Design review of the part built by this model. Coordinates are the model's own, in mm. Give positions to 0.01 mm unless a question says otherwise; leave off trailing zeros. Write each loop counter-clockwise with the first axis right and the second up, starting at its lowest first coordinate (ties: lowest second). Pieces come first, ordered by that corner, then holes. Notation, with made-up numbers: (83.5, 62.25) -> (140.5, 62.25) arc R20 ccw to (140.5, 79.25) -> close; hole circle Ø3 at (-36.5, 32.5). An arc over 180 degrees is marked (long way). Use CSV: the item, a comma, the result in double quotes.
Autodesk Inventor part; units mm, degrees
ref_plane "Work Plane1" through (167.5, 74.771, 0) normal (0.7444, -0.6677, 0) x (0.6677, 0.7444, 0)
ref_plane "Work Plane2" through (0, 0, 0) normal (0, -1, 0) x (1, 0, 0)
ref_plane "YZ Plane" through (0, 0, 0) normal (1, 0, 0) x (0, 1, 0)
sketch "Sketch1" plane through (0, 0, 0) normal (0, 0, 1) x (1, 0, 0)
  circle A0 centre (0, 225) radius 225 construction
  circle A1 centre (0, 225) radius 220 construction
  line L0 (0, 5) -> (0, 0)
  arc A2 (0, 0) -> (167.5, 74.771) centre (0, 225) ccw
  line L1 (167.5, 74.771) -> (163.7778, 78.1094)
  arc A3 (0, 5) -> (163.7778, 78.1094) centre (0, 225) ccw
  dimension "d0" = 450
  dimension "d1" = 5
  dimension "d2" = 5
  dimension "d3" = 167.5
extrude "Extrusion1" add sketch "Sketch1" along normal blind 75
ref_plane "Work Plane1" through (167.5, 74.771, 0) normal (0.7444, -0.6677, 0) x (0.6677, 0.7444, 0)
sketch "Sketch2" plane through (167.5, 74.771, 0) normal (0.7444, -0.6677, 0) x (0.6677, 0.7444, 0)
  circle A0 centre (-5, 47.5) radius 3
  circle A1 centre (-5, 27.5) radius 3
  line L0 (0, 0) -> (-167.5, 0)
  line L1 (0, 0) -> (0, 75)
  line L2 (-167.5, 75) -> (0, 75)
  line L3 (-167.5, 0) -> (-167.5, 75)
  dimension "d6" = 6
  dimension "d7" = 6
  dimension "d8" = 5
  dimension "d9" = 27.5
  dimension "d10" = 20
extrude "Extrusion2" cut sketch "Sketch2" along normal through all both and the other way through all contours A0 | A1
ref_plane "Work Plane2" through (0, 0, 0) normal (0, -1, 0) x (1, 0, 0)
sketch "Sketch3" plane through (0, 0, 0) normal (0, -1, 0) x (1, 0, 0)
  circle A0 centre (5, 47.5) radius 3
  circle A1 centre (5, 27.5) radius 3
  circle A2 centre (55, 47.5) radius 3
  circle A3 centre (55, 27.5) radius 3
  circle A4 centre (65.5, 47.5) radius 3
  circle A5 centre (65.5, 27.5) radius 3
  point P0 (0, 0)
  dimension "d13" = 6
  dimension "d14" = 6
  dimension "d15" = 6
  dimension "d16" = 6
  dimension "d17" = 27.5
  dimension "d18" = 20
  dimension "d19" = 5
  dimension "d20" = 55
  dimension "d23" = 6
  dimension "d24" = 6
  dimension "d25" = 10.5
extrude "Extrusion3" cut sketch "Sketch3" along normal through all both and the other way through all
properties part number "CW004" material "ABS Plastic"
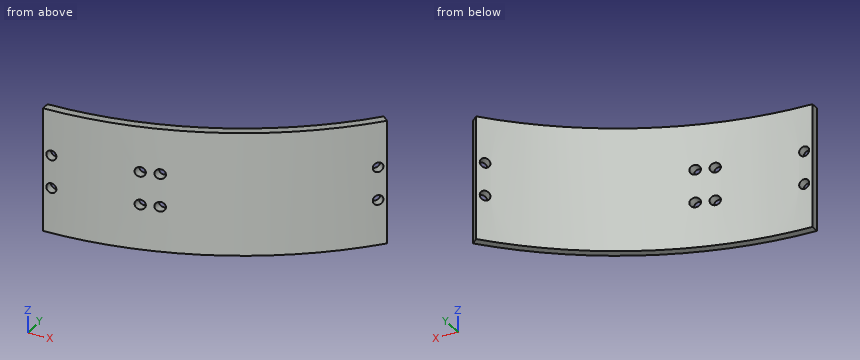
(1) Take a section at D-D (x = 5). Write out the cut boundary in (y, z).
Established:
outline,"(0.06, 0) -> (5.06, 0) -> (5.06, 24.5) -> (0.06, 24.5) -> close; (0.06, 30.5) -> (5.06, 30.5) -> (5.06, 44.5) -> (0.06, 44.5) -> close; (0.06, 50.5) -> (5.06, 50.5) -> (5.06, 75) -> (0.06, 75) -> close"
(2) For line 1 along Z through (x, y) = (65.5, 10.5); line 2 along X through (y, z) = (27, 48.5); line 3 along Y through (x, z) = (70, 52), list the stretches that pass through material, from the lowest coordinate up. Write a range as [from, to].
Established:
line 1,"z = [0, 24.5], [30.5, 44.5], [50.5, 75]"
line 2,"x = [95.9, 106.87]"
line 3,"y = [11.17, 16.43]"
(3) Take a section at A-A (x = 65.5). Write out the cut boundary in (y, z), then the cut area to 3 significant figures.
Established:
outline,"(9.74, 0) -> (14.98, 0) -> (14.98, 24.5) -> (9.74, 24.5) -> close; (9.74, 30.5) -> (14.98, 30.5) -> (14.98, 44.5) -> (9.74, 44.5) -> close; (9.74, 50.5) -> (14.98, 50.5) -> (14.98, 75) -> (9.74, 75) -> close"
area,"330 mm2"
(4) Take a section at C-C (z = 17). Write out the cut boundary in (x, y), then the cut area to 3 significant figures.
Established:
outline,"(0, 0) arc R225 ccw to (167.5, 74.77) -> (163.78, 78.11) arc R220 cw to (0, 5) -> close"
area,"934 mm2"
(5) Take a section at B-B (z = 27.5). Write out the cut boundary in (x, y).
Established:
outline,"(0, 0) arc R225 ccw to (2, 0.01) -> (2, 5.01) arc R220 cw to (0, 5) -> close; (8, 0.14) arc R225 ccw to (52, 6.09) -> (52, 11.23) arc R220 cw to (8, 5.15) -> close; (58, 7.6) arc R225 ccw to (62.5, 8.85) -> (62.5, 14.06) arc R220 cw to (58, 12.78) -> close; (68.5, 10.68) arc R225 ccw to (162.05, 68.91) -> (158.33, 72.25) arc R220 cw to (68.5, 15.94) -> close; (162.44, 76.63) -> (166.16, 73.29) arc R225 ccw to (167.5, 74.77) -> (163.78, 78.11) arc R220 cw to start"
(6) Clearance check with flat-ended pins moving along their axes: pin 1 (12 mm diameter, centred on y = 17.5, z = 17, fed in from +X); pin 2 (8 mm diameter, centred on x = 55, z = 27.5, fed in from +Y); pin 3 (8 mm diameter, centred on x = 65.5, z = 27.5, fed in from -Y). State where each tip first meets the part, or that it passes through.
Established:
pin 1,"stops at x = 100.11"
pin 2,"stops at y = 13.06"
pin 3,"stops at y = 8.57"
